Check sheet for the drawn part. Datum: minimum x, y, z corner. Units: mm. A direction names the side the tool comes from. Give positions to 0.01 mm unless a question says otherwise; leave off trailing zeros. Write each loop counter-clockwise with the first axis right and the second up, starting at its lowest first coordinate (ties: lowest second). Pieces come first, ordered by that corner, then holes. Notation, with made-up numbers: M 15,-0.75 L 46,-0.75 A24 ccw 46,34.25 Z; hole C 49.5,31 d9. An arc over 180 degrees is marked long. Write item = value, one per line. Start each with the question number.
1) Draft check along Y on the marked faces 3, 4, 5 and 6. Enter one of: pulls with the +Y half, pulls with the -Y half, needs draft (parallel to the pull), parting line crosses it, or undercut.
2) Set-up check for the marked faces 1 and 2: record each of +Z, -Z, +X, -X, +Y, -Y from which the full face is reachable in a straight line by a thin tool's end or side.
3) Sectioned sample at B-B, the plane x = 10. Record the cut outline in (y, z).
4) Sectioned sample at D-D, the plane z = 2.5. Record the cut outline in (x, y).
5) Scan lines: L1, parallel to X at y = 21, z = 11; L2, parallel to Y at x = 10, z = 18.55; L3, parallel to X at y = 16.5, z = 19.35. Record each from-to range of solid material in increasing order.
6) Sectioned sample at C-C, the plane z = 15. Record the cut outline in (x, y).
7) Sectioned sample at A-A, the plane y = 16.5. Record the cut outline in (x, z).
8) Gauge pin test, flat ends, axial feed: pin 1 (1 mm diameter, centred on x = 10, y = 32, fed in from -Z); pin 2 (9 mm diameter, centred on x = 10, y = 16.5, fed in from -Z). Record the tip position at first contact, or that the pin passes through.
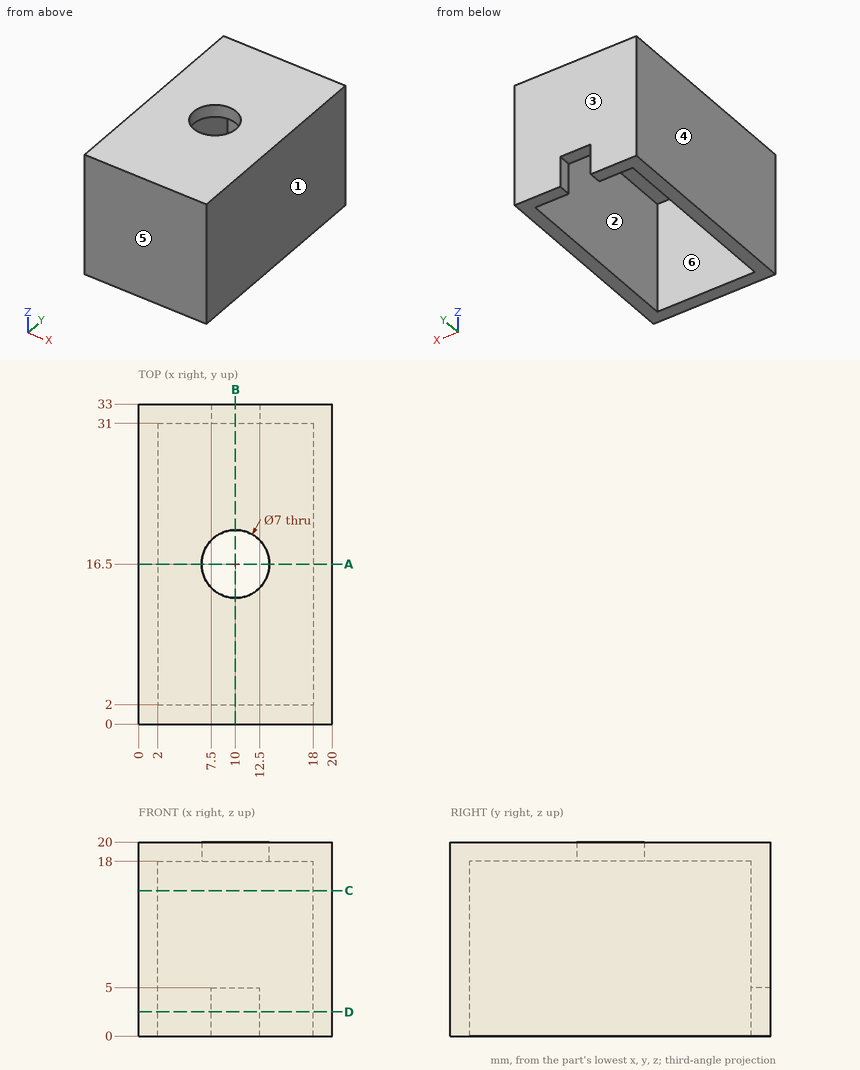
Data:
q1.face_3 = pulls with the +Y half
q1.face_4 = needs draft
q1.face_5 = pulls with the -Y half
q1.face_6 = undercut
q2.face_1 = +Z, -Z, +X, +Y, -Y
q2.face_2 = -Z
q3.outline = M 0,0 L 2,0 L 2,18 L 13,18 L 13,20 L 0,20 Z; M 20,18 L 31,18 L 31,5 L 33,5 L 33,20 L 20,20 Z
q4.outline = M 0,0 L 20,0 L 20,33 L 12.5,33 L 12.5,31 L 18,31 L 18,2 L 2,2 L 2,31 L 7.5,31 L 7.5,33 L 0,33 Z
q5.L1 = 0 to 2, 18 to 20
q5.L2 = 0 to 13, 20 to 33
q5.L3 = 0 to 6.5, 13.5 to 20
q6.outline = M 0,0 L 20,0 L 20,33 L 0,33 Z; hole M 2,2 L 18,2 L 18,31 L 2,31 Z
q7.outline = M 0,0 L 2,0 L 2,18 L 6.5,18 L 6.5,20 L 0,20 Z; M 13.5,18 L 18,18 L 18,0 L 20,0 L 20,20 L 13.5,20 Z
q8.pin_1 = 5
q8.pin_2 = 18
